Input: part model. Units: mm. Frame: model coordinates. Face numbers are marked on the shaded views. Round coordinates to 2 decimals unless told otherwise and drop trailing zeros. Loops run counter-clockwise (first coordinate to the right, second up) from the corner with the lowest first, then second, coordinate; pieces in that order, holes last.
1) Section A-A, the plane y = 0. State how many separate pieces and enclosed holes the cut face has, and give its area (3 significant figures).
2) First-contact query: pin 1 (10 mm diameter, centred on x = 353.5, y = 33.5, fed in from -Z); pin 2 (8 mm diameter, centred on x = 446.5, y = 57.5, fed in from -Z). Flat tips, straight axial feed; report the tip coordinate or a pass-through.
3) Section D-D, the plane x = -81. Return loops of the section in (y, z), and give its area (3 significant figures).
4) Draft query along Y for the marked faces 1, 2, 3 and 4. Return one class per face: pulls with the +Y half, pulls with the -Y half, needs draft (parallel to the pull), parting line crosses it, or undercut.
5) Section C-C, the plane x = 469.9. Return loops of the section in (y, z).
6) Section B-B, the plane z = -12.5. Return loops of the section in (x, y), and give its area (3 significant figures).
7) Ray query, line 1 along Z through (x, y) = (405.5, 4.5); line 2 along Y through (x, z) = (-414.5, 21); line 3 along Y through (x, z) = (138, -9.5). Return the intervals inside material, ascending.
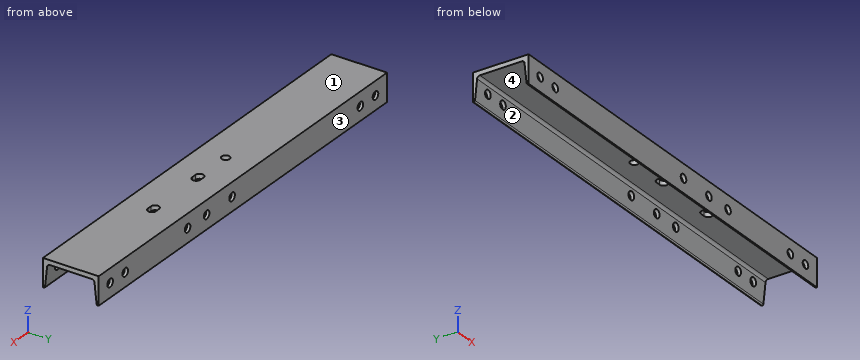
from build123d import *

# Parameters (mm, degrees)
BOSS_EXTRUDE1_DEPTH = 576.2625
SKETCH5_R           = 11.1125
CUT_EXTRUDE3_DEPTH  = 152.4
SKETCH6_R           = 11.1125
CUT_EXTRUDE4_DEPTH  = 13.7


with BuildPart() as part:
    # Sketch1 → Boss-Extrude1 (new body, symmetric)
    with BuildSketch(Plane(origin=(0, 0, 0), x_dir=(0, 0, -1), z_dir=(1, 0, 0))):
        with BuildLine():
            Line((-48.8061, -76.2), (-48.8061, 76.2))
            Line((-48.8061, 76.2), (27.3939, 76.2))
            Line((27.3939, 76.2), (27.3939, 73.710744653))
            ThreePointArc((27.3939, 73.710744653), (26.61173954, 71.672050174), (24.666685315, 70.679672107))
            Line((24.666685315, 70.679672107), (-29.288063286, 64.969518115))
            ThreePointArc((-29.288063286, 64.969518115), (-34.150698849, 62.488572947), (-36.1061, 57.391836749))
            Line((-36.1061, 57.391836749), (-36.1061, -57.391836749))
            ThreePointArc((-36.1061, -57.391836749), (-34.150698849, -62.488572947), (-29.288063286, -64.969518115))
            Line((-29.288063286, -64.969518115), (24.666685315, -70.679672107))
            ThreePointArc((24.666685315, -70.679672107), (26.61173954, -71.672050174), (27.3939, -73.710744653))
            Line((27.3939, -73.710744653), (27.3939, -76.2))
            Line((27.3939, -76.2), (-48.8061, -76.2))
        make_face()
    extrude(amount=BOSS_EXTRUDE1_DEPTH, both=True)

    # Sketch5 → Cut-Extrude3 (cut)
    with BuildSketch(Plane.XZ.offset(76.2)):
        with Locations((530.225, 10.7061)):
            Circle(SKETCH5_R)
        with Locations((469.9, 10.7061)):
            Circle(SKETCH5_R)
        with Locations((42.799, 10.7061)):
            Circle(SKETCH5_R)
        with Locations((220.599, 10.7061)):
            Circle(SKETCH5_R)
        with Locations((144.399, 10.7061)):
            Circle(SKETCH5_R)
        with Locations((-530.225, 10.7061)):
            Circle(SKETCH5_R)
        with Locations((-469.9, 10.7061)):
            Circle(SKETCH5_R)
    extrude(amount=-CUT_EXTRUDE3_DEPTH, mode=Mode.SUBTRACT)

    # Sketch6 → Cut-Extrude4 (cut, through all)
    with BuildSketch(Plane(origin=(0, 0, 36.1061), x_dir=(-1, 0, 0), z_dir=(0, 0, -1))):
        with Locations((42.8625, 0)):
            Circle(SKETCH6_R)
        with BuildLine():
            Line((-74.6125, 11.1125), (-61.9125, 11.1125))
            ThreePointArc((-61.9125, 11.1125), (-50.8, 0), (-61.9125, -11.1125))
            Line((-61.9125, -11.1125), (-74.6125, -11.1125))
            ThreePointArc((-74.6125, -11.1125), (-85.725, 0), (-74.6125, 11.1125))
        make_face()
        with BuildLine():
            Line((-239.7125, -11.1125), (-252.4125, -11.1125))
            ThreePointArc((-252.4125, -11.1125), (-263.525, 0), (-252.4125, 11.1125))
            Line((-252.4125, 11.1125), (-239.7125, 11.1125))
            ThreePointArc((-239.7125, 11.1125), (-228.6, 0), (-239.7125, -11.1125))
        make_face()
    extrude(amount=-CUT_EXTRUDE4_DEPTH, mode=Mode.SUBTRACT)


solid = part.part
Final values:
1. separate pieces: 4
1. enclosed holes: 0
1. area: 13,500 mm2
2. pin 1: stops at z = 36.11
2. pin 2: stops at z = 34.9
3. outline: (-76.2, -27.39) - (-73.71, -27.39) arc R3.05 ccw to (-70.68, -24.67) - (-64.97, 29.29) arc R7.62 cw to (-57.39, 36.11) - (57.39, 36.11) arc R7.62 cw to (64.97, 29.29) - (70.68, -24.67) arc R3.05 ccw to (73.71, -27.39) - (76.2, -27.39) - (76.2, 48.81) - (-76.2, 48.81) - close
3. area: 3,040 mm2
4. face 1: needs draft
4. face 2: undercut
4. face 3: pulls with the +Y half
4. face 4: undercut
5. outline: (-76.2, -27.39) - (-73.71, -27.39) arc R3.05 ccw to (-70.68, -24.67) - (-68.11, -0.41) - (-76.2, -0.41) - close; (-76.2, 21.82) - (-65.76, 21.82) - (-64.97, 29.29) arc R7.62 cw to (-57.39, 36.11) - (57.39, 36.11) arc R7.62 cw to (64.97, 29.29) - (65.76, 21.82) - (76.2, 21.82) - (76.2, 48.81) - (-76.2, 48.81) - close; (68.11, -0.41) - (70.68, -24.67) arc R3.05 ccw to (73.71, -27.39) - (76.2, -27.39) - (76.2, -0.41) - close
6. outline: (-576.26, -76.2) - (576.26, -76.2) - (576.26, -69.39) - (-576.26, -69.39) - close; (-576.26, 69.39) - (576.26, 69.39) - (576.26, 76.2) - (-576.26, 76.2) - close
6. area: 15,700 mm2
7. line 1: z = 36.11 to 48.81
7. line 2: y = -76.2 to -65.85, 65.85 to 76.2
7. line 3: y = -76.2 to -69.07, 69.07 to 76.2
